Here's the drawing with two shaded views (mm, measured from the low corner). I have some questions. Round coordinates to 2 decimals unless told otherwise and drop trailing zeros. Order: outer loops, then holes, each group sorted by start corner. A loop starts at its lowest first (then second) coordinate and runs counter-clockwise, first axis right, second up. Notation, with made-up numbers: (37, 46.5) -> (86, 46.5) arc R22 cw to (86, 61.5) -> close; hole circle Ø7 at (60, -3). An arc over 180 degrees is marked (long way). One line per question, with ' | ' between items.
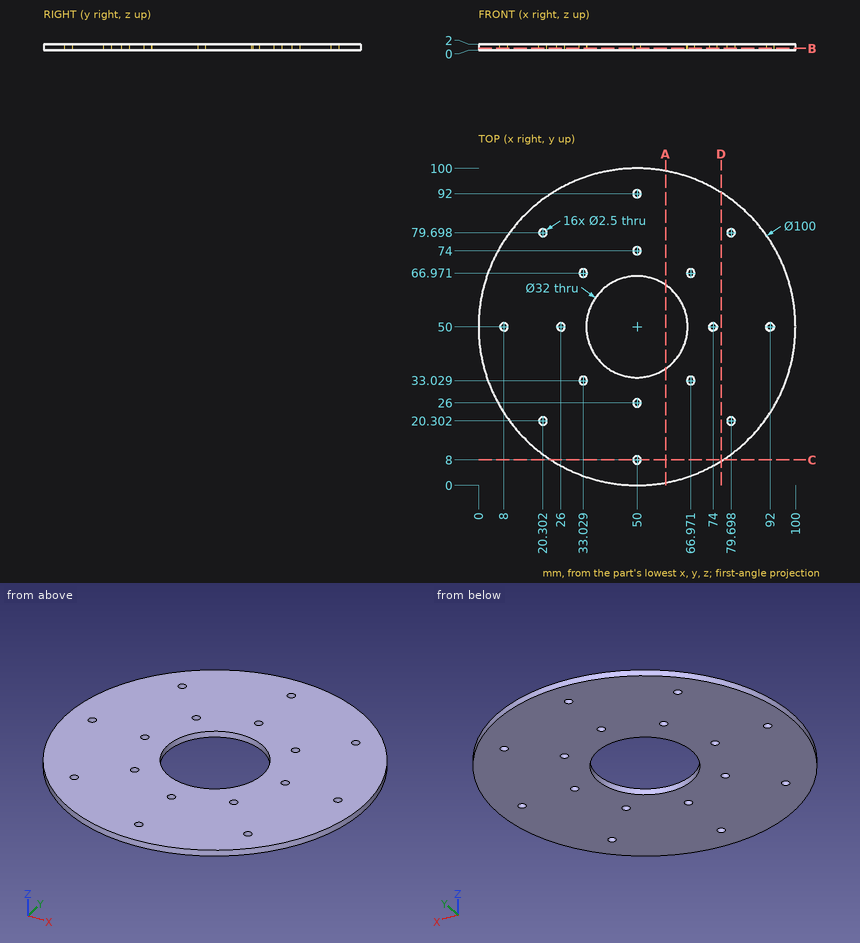
1. I want a section at D-D on x = 76.5. List the corners of the cut face in (y, z) for me.
From the geometry:
outline: (7.6, 0) -> (92.4, 0) -> (92.4, 2) -> (7.6, 2) -> close
2. I want a section at C-C on y = 8. List the corners of the cut face in (x, z) for me.
From the geometry:
outline: (22.87, 0) -> (48.75, 0) -> (48.75, 2) -> (22.87, 2) -> close; (51.25, 0) -> (77.13, 0) -> (77.13, 2) -> (51.25, 2) -> close
3. I want a section at A-A on x = 59. List the corners of the cut face in (y, z) for me, and give its area (3 significant figures).
From the geometry:
outline: (0.82, 0) -> (36.77, 0) -> (36.77, 2) -> (0.82, 2) -> close; (63.23, 0) -> (99.18, 0) -> (99.18, 2) -> (63.23, 2) -> close | area: 144 mm²
4. I want a section at B-B on z = 0.6. Count the separate pieces of the cut face and the enclosed holes in it, and give its area (3 significant figures).
From the geometry:
separate pieces: 1 | enclosed holes: 17 | area: 6,970 mm²
5. I need wall thicknesses on probe 1 along X at (y, z) = (49.5, 1.8) (1 decimal); probe 2 along X at (y, z) = (59, 0.5) (1 decimal); probe 3 along X at (y, z) = (80.5, 0.9). Which ranges of each line are inside material? Lowest first, please.
From the geometry:
probe 1: x = 0 to 6.9, 9.1 to 24.9, 27.1 to 34, 66 to 72.9, 75.1 to 90.9, 93.1 to 100 | probe 2: x = 0.8 to 36.8, 63.2 to 99.2 | probe 3: x = 10.38 to 19.34, 21.26 to 78.74, 80.66 to 89.62
6. I'm going to push flat-ended pins straight in: pin 1 (2 mm diameter, centred on x = 66.97, y = 66.97, fed in from -Z); pin 2 (1 mm diameter, centred on y = 82.5, z = 0, fed in from -X). Where does each tip first touch, or does it pass through?
From the geometry:
pin 1: passes through | pin 2: stops at x = 11.58
